from build123d import *

# Parameters (mm, degrees)
EXTRUDE1_DEPTH     = 19.685
CHAMFER1_SIZE      = 3.302
FILLET1_R          = 0.762
SKETCH2_W          = 17.907
SKETCH2_H          = 2.54
EXTRUDE2_DEPTH     = 7.493
SKETCH4_W          = 17.907
SKETCH4_H          = 2.54
EXTRUDE3_DEPTH     = 7.493
FILLET2_R          = 0.762
EXTRUDE4_DEPTH     = 36.35375
SKETCH10_R         = 2.159
CUT_EXTRUDE1_DEPTH = 36.35375
SKETCH19_R         = 2.159
CUT_EXTRUDE2_DEPTH = 59.72110295
RIB2_START         = -0.6985
RIB2_DEPTH         = 1.397
RIB3_START         = -0.6985
RIB3_DEPTH         = 1.397
SKETCH16_R         = 5.0165
EXTRUDE5_DEPTH     = 1.651
SKETCH18_R         = 4.953
EXTRUDE6_DEPTH     = 0.127
SKETCH20_R         = 2.8575
SKETCH20_R_2       = 1.27
EXTRUDE7_DEPTH     = 4.064
SKETCH22_W         = 5.715
SKETCH22_H         = 3.175
EXTRUDE8_DEPTH     = 1.905
SKETCH24_R         = 0.635


with BuildPart() as part:
    # Sketch1 → Extrude1 (new body)
    with BuildSketch(Plane.XY):
        Polygon((0, 0), (40.2, 0), (40.2, 31.59125), (20.6375, 35.56), (0, 35.56), align=None)
    extrude(amount=EXTRUDE1_DEPTH)

    # Chamfer1
    chamfer1_edges = [part.edges().sort_by_distance(p)[0] for p in [
        (0, 35.56, 9.8425),
    ]]
    chamfer(chamfer1_edges, length=CHAMFER1_SIZE)

    # Fillet1
    fillet1_edges = [part.edges().sort_by_distance(p)[0] for p in [
        (20.1, 0, 0),
        (20.1, 0, 19.685),
        (40.2, 0, 9.8425),
        (0, 0, 9.8425),
    ]]
    fillet(fillet1_edges, radius=FILLET1_R)

    # Sketch2 → Extrude2 (add)
    with BuildSketch(Plane(origin=(40.2, 0, 0), x_dir=(0, 0, -1), z_dir=(1, 0, 0))):
        with Locations((-9.8425, 26.76525)):
            Rectangle(SKETCH2_W, SKETCH2_H)
    extrude(amount=EXTRUDE2_DEPTH)

    # Sketch4 → Extrude3 (add)
    with BuildSketch(Plane.ZY):
        with Locations((9.8425, 26.76652)):
            Rectangle(SKETCH4_W, SKETCH4_H)
    extrude(amount=EXTRUDE3_DEPTH)

    # Fillet2
    fillet2_edges = [part.edges().sort_by_distance(p)[0] for p in [
        (47.693, 26.76525, 18.796),
        (47.693, 26.76525, 0.889),
        (-7.493, 26.76652, 0.889),
        (-7.493, 26.76652, 18.796),
    ]]
    fillet(fillet2_edges, radius=FILLET2_R)

    # Sketch5 → Extrude4 (add)
    with BuildSketch(Plane(origin=(0, 0, 0), x_dir=(1, 0, 0), z_dir=(0, 1, 0))):
        with BuildLine():
            Line((1.143, -0.837535442), (20.828, -0.837535442))
            Line((20.828, -0.837535442), (20.828, -7.022435442))
            ThreePointArc((20.828, -7.022435442), (18.034, -9.816435442), (20.828, -12.610435442))
            Line((20.828, -12.610435442), (20.828, -18.795335442))
            Line((20.828, -18.795335442), (1.143, -18.795335442))
            Line((1.143, -18.795335442), (1.143, -0.837535442))
        make_face()
    extrude(amount=EXTRUDE4_DEPTH)

    # Loft1: read off the stored shape, not the designer's step
    # Loft1: loft between two sections, ruled curve by curve
    loft1_from = [
        Edge.make_bspline([(21.641638875, 35.356284925, 7.777844123), (20.350474841, 35.618230344, 7.645115734), (19.387970871, 35.813498721, 8.533256016), (19.387970871, 35.813498721, 11.181528503), (20.350474841, 35.618230344, 12.069668784), (21.641638875, 35.356284925, 11.936940395)], [0, 0, 0, 0, 0.5, 0.5, 1, 1, 1, 1], 3, [1, 0.609161307, 0.475443008, 0.475443008, 0.609161307, 1]),
        Edge.make_bspline([(21.641638875, 35.356284925, 18.877249077), (36.963924395, 32.247770131, 18.877249077)], [0, 0, 1, 1], 1),
        Edge.make_line((21.641638875, 35.356284925, 0.837535442), (36.963924395, 32.247770131, 0.837535442)),
        Edge.make_line((36.963924395, 32.247770131, 0.837535442), (36.963924395, 32.247770131, 18.877249077)),
        Edge.make_line((21.641638875, 35.356284925, 7.777844123), (21.641638875, 35.356284925, 0.837535442)),
        Edge.make_line((21.641638875, 35.356284925, 18.877249077), (21.641638875, 35.356284925, 11.936940395)),
    ]
    loft1_to = [
        Edge.make_bspline([(21.844, 36.35375, 7.720935442), (20.79625, 36.35375, 7.720935442), (19.7485, 36.35375, 8.419435442), (19.7485, 36.35375, 11.213435442), (20.79625, 36.35375, 11.911935442), (21.844, 36.35375, 11.911935442)], [0, 0, 0, 0, 0.5, 0.5, 1, 1, 1, 1], 3, [1, 0.666666667, 0.5, 0.5, 0.666666667, 1]),
        Edge.make_bspline([(21.844, 36.35375, 18.795335442), (34.544, 36.35375, 18.795335442)], [0, 0, 1, 1], 1),
        Edge.make_line((21.844, 36.35375, 0.837535442), (34.544, 36.35375, 0.837535442)),
        Edge.make_line((34.544, 36.35375, 0.837535442), (34.544, 36.35375, 18.795335442)),
        Edge.make_line((21.844, 36.35375, 7.720935442), (21.844, 36.35375, 0.837535442)),
        Edge.make_line((21.844, 36.35375, 18.795335442), (21.844, 36.35375, 11.911935442)),
    ]
    loft1 = Solid(Shell([*[Face.make_surface_from_curves(loft1_from[k], loft1_to[k]) for k in range(6)], Face(Wire(loft1_from)), Face(Wire(loft1_to))]))
    add(loft1)

    # Sketch10 → Cut-Extrude1 (cut)
    with BuildSketch(Plane(origin=(0, 28.03525, 0), x_dir=(-1, 0, 0), z_dir=(0, 1, 0))):
        with Locations(Location((-44.264, 4.699, 0), (0, 0, 90))):
            Circle(SKETCH10_R)
        with Locations(Location((-44.264, 14.986, 0), (0, 0, 90))):
            Circle(SKETCH10_R)
    extrude(amount=-CUT_EXTRUDE1_DEPTH, mode=Mode.SUBTRACT)

    # Sketch19 → Cut-Extrude2 (cut, through all)
    with BuildSketch(Plane(origin=(0, 28.03652, 0), x_dir=(-1, 0, 0), z_dir=(0, 1, 0))):
        with Locations(Location((4.064, 4.699, 0), (0, 0, 90))):
            Circle(SKETCH19_R)
        with Locations(Location((4.064, 14.986, 0), (0, 0, 90))):
            Circle(SKETCH19_R)
    extrude(amount=-CUT_EXTRUDE2_DEPTH, mode=Mode.SUBTRACT)

    # Rib2: read off the stored shape, not the designer's step
    # Rib2 outline → Rib2 (add)
    with BuildSketch(Plane.XY.offset(9.8425).offset(RIB2_START)):
        Polygon((43.95, 28.03525), (43.2, 28.78525), (40.2, 29.53525), (40.2, 28.03525), align=None)
    extrude(amount=RIB2_DEPTH)

    # Rib3: read off the stored shape, not the designer's step
    # Rib3 outline → Rib3 (add)
    with BuildSketch(Plane.XY.offset(9.8425).offset(RIB3_START)):
        Polygon((0, 29.53652), (-3, 28.78652), (-3.75, 28.03652), (0, 28.03652), align=None)
    extrude(amount=RIB3_DEPTH)

    # Sketch16 → Extrude5 (add)
    with BuildSketch(Plane(origin=(0, 36.35375, 0), x_dir=(-1, 0, 0), z_dir=(0, 1, 0))):
        with Locations(Location((-10, 9.8425, 0), (0, 0, 270))):
            Circle(SKETCH16_R)
    extrude(amount=EXTRUDE5_DEPTH)

    # Loft2: read off the stored shape, not the designer's step
    # Loft2: loft between two sections, ruled curve by curve
    loft2_from = [
        Edge.make_bspline([(10.789313033, 36.35375, 2.774435984), (-3.346815, 36.35375, 1.195809919), (-4.925441065, 36.35375, 15.331937951), (9.210686967, 36.35375, 16.910564016), (23.346815, 36.35375, 18.489190081), (24.925441065, 36.35375, 4.353062049), (10.789313033, 36.35375, 2.774435984)], [0, 0, 0, 0, 0.5, 0.5, 0.5, 1, 1, 1, 1], 3, [1, 0.333333333, 0.333333333, 1, 0.333333333, 0.333333333, 1]),
    ]
    loft2_to = [
        Edge.make_bspline([(9.493399511, 38.00475, 4.851645545), (-0.488309399, 38.00475, 5.864846522), (0.524891578, 38.00475, 15.846555433), (10.506600489, 38.00475, 14.833354455), (20.488309399, 38.00475, 13.820153478), (19.475108422, 38.00475, 3.838444567), (9.493399511, 38.00475, 4.851645545)], [0, 0, 0, 0, 0.5, 0.5, 0.5, 1, 1, 1, 1], 3, [1, 0.333333333, 0.333333333, 1, 0.333333333, 0.333333333, 1]),
    ]
    loft2 = Solid(Shell([*[Face.make_surface_from_curves(loft2_from[k], loft2_to[k]) for k in range(1)], Face(Wire(loft2_from)), Face(Wire(loft2_to))]))
    add(loft2)

    # Sketch18 → Extrude6 (add)
    with BuildSketch(Plane(origin=(0, 38.00475, 0), x_dir=(-1, 0, 0), z_dir=(0, 1, 0))):
        with Locations(Location((-10, 9.8425, 0), (0, 0, 90))):
            Circle(SKETCH18_R)
    extrude(amount=EXTRUDE6_DEPTH)

    # Sketch20 → Extrude7 (add)
    with BuildSketch(Plane(origin=(0, 38.13175, 0), x_dir=(-1, 0, 0), z_dir=(0, 1, 0))):
        with Locations(Location((-10, 9.8425, 0), (0, 0, 90))):
            Circle(SKETCH20_R)
        with Locations(Location((-10, 9.8425, 0), (0, 0, 90))):
            Circle(SKETCH20_R_2, mode=Mode.SUBTRACT)
    extrude(amount=EXTRUDE7_DEPTH)

    # Sketch22 → Extrude8 (add)
    with BuildSketch(Plane.ZY):
        with Locations((9.8425, 2.8575)):
            Rectangle(SKETCH22_W, SKETCH22_H)
    extrude(amount=EXTRUDE8_DEPTH)

    # Sketch21 → section 0 of loft3
    with BuildSketch(Plane.ZY, mode=Mode.PRIVATE) as loft3_s0:
        with BuildLine():
            Line((6.477, 4.953), (13.208, 4.953))
            Line((13.208, 4.953), (13.208, 0.762))
            Line((13.208, 0.762), (6.477, 0.762))
            Line((6.477, 0.762), (6.477, 4.953))
        make_face()
    # loft up to a face of the part (loft3)
    loft([loft3_s0.sketch, part.faces().sort_by_distance((-1.905, 2.8575, 9.8425))[0]])

    # Sweep3: sweep along a path in Sketch23
    with BuildLine(Plane.XY.offset(9.8425)) as sweep3_path:
        ThreePointArc((-1.905, 2.946484605), (-3.908218654, 2.753050744), (-5.763136487, 1.972293764))
    # Sketch24 → Sweep3 (sweep)
    with BuildSketch(Plane.ZY.offset(1.905)):
        with Locations((9.8425, 2.946484605)):
            Circle(SKETCH24_R)
        with Locations((11.23883905, 2.946484605)):
            Circle(SKETCH24_R)
        with Locations((8.466018651, 2.946484605)):
            Circle(SKETCH24_R)
    sweep(path=sweep3_path.line)


solid = part.part
Could you check a few things on this model? Use its own coordinates, in mm. A direction names the side the tool comes from. Coordinates: 2 decimals unless noted, no trailing zeros. Order: outer loops, then holes, each group sorted by start corner. A loop starts at its lowest first (then second) coordinate and runs counter-clockwise, first axis right, second up.
Q1. Will these pins go through, and if not, where does the flat tip stop? pin 1 (8 mm diameter, centred on x = 42.5, z = 6.5, fed in from +Y); pin 2 (10 mm diameter, centred on x = 41, z = 12.5, fed in from +Y); pin 3 (2 mm diameter, centred on x = 18.5, z = 12, fed in from +Y).
Q2. Suppose I cut it at A-A on y = 14. Please give me the cut outline in (x, z) (3 decimals), and give its area (3 significant figures).
Q3. Suppose I cut it at B-B on z = 4. Give the number of separate pieces and of enclosed holes in the cut face, and give its area (3 significant figures).
Q4. Thinking about a two-plate mould opening in X: for faces 5 (the flat face through (9, 42.196, 11)), 6 (the flat face through (-7.493, 27, 10)), 7 (the flat face through (10, 38.132, 10)), which applies, released by +X, released by -X, zero draft, split by the parting line, or undercut?
Q5. Which directions (+Z, -Z, +X, -X, +Y, -Y) give clear straight access to the entire face, cutting with the end or side of a thin tool? Please do faces 1 (the flat face through (44, 25.495, 10)), 2 (the flat face through (41.6, 28.6, 10.541)), 3 (the flat face through (-1, 29, 9.144)), 4 (the flat face through (19.6, 35.56, 9.8)).
Q6. Please list where these lines run through material, in increasing order: L1, parallel to X at y = 28, z = 14.75; L2, parallel to Y at x = 3, z = 14; L3, parallel to X at y = 17, z = 17.
Answer:
1. pin 1: stops at y = 31.94
1. pin 2: stops at y = 33.88
1. pin 3: stops at y = 36.35
2. outline: (0, 0) - (40.2, 0) - (40.2, 19.685) - (0, 19.685) - close
2. area: 791 mm2
3. separate pieces: 3
3. enclosed holes: 0
3. area: 1,460 mm2
4. face 5: zero draft
4. face 6: released by -X
4. face 7: undercut
5. face 1: +Z, -Z, +X, -Y
5. face 2: +Z, +X, +Y
5. face 3: -Z, -X, +Y
5. face 4: none
6. L1: x = -7.49 to -6.21, -1.92 to 42.12, 46.41 to 47.69
6. L2: y = 0 to 36.35
6. L3: x = 0 to 40.2
